```python
from build123d import *

# Parameters (mm, degrees)
SKETCH3_W                                       = 50
SKETCH3_H                                       = 50
BOSS_EXTRUDE1_DEPTH                             = 8
SKETCH3_3_R                                     = 1.5
SKETCH3_3_R_2                                   = 8
CUT_EXTRUDE2_DEPTH                              = 10
SKETCH4_R                                       = 18.5
CUT_EXTRUDE3_DEPTH                              = 4
BOSS_EXTRUDE2_DEPTH                             = 15
BOSS_EXTRUDE2_DEPTH_BACK                        = 23
SKETCH6_W                                       = 80
SKETCH6_H                                       = 5
CSK_FOR_M3_FLAT_HEAD_MACHINE_SCREW1_D           = 3.4
CSK_FOR_M3_FLAT_HEAD_MACHINE_SCREW1_CSINK_D     = 6.3
CSK_FOR_M3_FLAT_HEAD_MACHINE_SCREW1_CSINK_ANGLE = 90
SKETCH11_R                                      = 6.207
SKETCH11_R_2                                    = 5.207
BOSS_EXTRUDE3_DEPTH                             = 5


with BuildPart() as part:
    # Sketch3 → Boss-Extrude1 (new body)
    with BuildSketch(Plane.XY):
        with Locations((0, 25)):
            Rectangle(SKETCH3_W, SKETCH3_H)
    extrude(amount=BOSS_EXTRUDE1_DEPTH)

    # Sketch3_3 → Cut-Extrude2 (cut)
    with BuildSketch(Plane.XY):
        with Locations(Location((-7.75, 38.423393759, 0), (0, 0, 180))):
            Circle(SKETCH3_3_R)
        with Locations(Location((7.75, 38.423393759, 0), (0, 0, 180))):
            Circle(SKETCH3_3_R)
        with Locations(Location((-7.75, 11.576606241, 0), (0, 0, 180))):
            Circle(SKETCH3_3_R)
        with Locations(Location((7.75, 11.576606241, 0), (0, 0, 180))):
            Circle(SKETCH3_3_R)
        with Locations(Location((15.5, 25, 0), (0, 0, 180))):
            Circle(SKETCH3_3_R)
        with Locations(Location((6.062177825, 28.499999999, 0), (0, 0, 180))):
            Circle(SKETCH3_3_R_2)
    extrude(amount=CUT_EXTRUDE2_DEPTH, mode=Mode.SUBTRACT)

    # Sketch4 → Cut-Extrude3 (cut)
    with BuildSketch(Plane.XY.offset(8)):
        with Locations((0, 25)):
            Circle(SKETCH4_R)
    extrude(amount=-CUT_EXTRUDE3_DEPTH, mode=Mode.SUBTRACT)

    # Sketch6 → Boss-Extrude2 (add, two sides: drawn at the far end of the back side and taken through both)
    with BuildSketch(Plane.XY.offset(8).offset(-BOSS_EXTRUDE2_DEPTH_BACK)):
        with Locations((0, 2.5)):
            Rectangle(SKETCH6_W, SKETCH6_H)
    extrude(amount=BOSS_EXTRUDE2_DEPTH + BOSS_EXTRUDE2_DEPTH_BACK)

    # CSK for M3 Flat Head Machine Screw1 (through all)
    with Locations(Plane(origin=(0, 5, 0), x_dir=(1, 0, 0), z_dir=(0, 1, 0))):
        with Locations((-32.5, 7.5), (-32.5, -15.5), (32.5, -15.5), (32.5, 7.5)):
            CounterSinkHole(CSK_FOR_M3_FLAT_HEAD_MACHINE_SCREW1_D / 2, CSK_FOR_M3_FLAT_HEAD_MACHINE_SCREW1_CSINK_D / 2, counter_sink_angle=CSK_FOR_M3_FLAT_HEAD_MACHINE_SCREW1_CSINK_ANGLE)

    # Sketch11 → Boss-Extrude3 (add)
    with BuildSketch(Plane(origin=(0, 0, 0), x_dir=(-1, 0, 0), z_dir=(0, 0, -1))):
        with Locations((17.917822175, 28.499999999)):
            Circle(SKETCH11_R)
        with Locations((17.917822175, 28.499999999)):
            Circle(SKETCH11_R_2, mode=Mode.SUBTRACT)
    extrude(amount=BOSS_EXTRUDE3_DEPTH)


solid = part.part
```
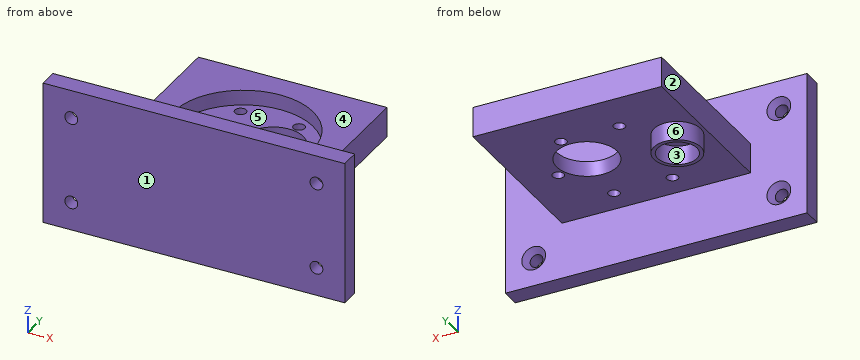
Input: part model. Units: mm. Frame: model coordinates. Face numbers are marked on the shaded views. A direction names the side the tool comes from. Round coordinates to 2 decimals unless told otherwise and drop trailing zeros. Loops run counter-clockwise (first coordinate to the right, second up) from the corner with the lowest first, then second, coordinate; pieces in that order, holes last.
1) Section query B-B on z = 1.5. Return the cut outline in (x, y).
Ans:
outline: (-40, 0) - (40, 0) - (40, 5) - (25, 5) - (25, 50) - (-25, 50) - (-25, 5) - (-40, 5) - close; hole circle Ø3 at (-7.75, 11.58); hole circle Ø3 at (-7.75, 38.42); hole circle Ø16 at (6.06, 28.5); hole circle Ø3 at (7.75, 11.58); hole circle Ø3 at (7.75, 38.42); hole circle Ø3 at (15.5, 25)
2) Pull-direction query (Y, two-part tool) for the marked faces 1, 2 and 3; classes: released by +Y, released by -Y, zero draft, split by the parting line, or undercut.
Ans:
face 1: released by -Y
face 2: zero draft
face 3: undercut
3) Section query C-C on y = 25. Return the cut outline in (x, z), plus the area to 3 significant figures.
Ans:
outline: (-25, 0) - (-23.04, 0) - (-23.04, -5) - (-21.77, -5) - (-21.77, 0) - (-14.06, 0) - (-14.06, -5) - (-12.79, -5) - (-12.79, 0) - (-1.13, 0) - (-1.13, 4) - (-18.5, 4) - (-18.5, 8) - (-25, 8) - close; (13.26, 0) - (14, 0) - (14, 4) - (13.26, 4) - close; (17, 0) - (25, 0) - (25, 8) - (18.5, 8) - (18.5, 4) - (17, 4) - close
area: 195 mm2
4) Pin query (flat end, axial travel): pin 1 (12 mm diameter, centred on y = 28.5, z = -6.5, fed in from +X); pin 2 (9 mm diameter, centred on y = 16.5, z = 2.5, fed in from +X); pin 3 (9.5 mm diameter, centred on x = -17.92, y = 28.5, fed in from -Z); pin 4 (2 mm diameter, centred on x = -32.5, z = 15.5, fed in from +Y). Return the tip coordinate at first contact, or that it passes through.
Ans:
pin 1: stops at x = -11.71
pin 2: stops at x = 25
pin 3: stops at z = 0
pin 4: passes through
5) Section query D-D on x = 7.75. Return the cut outline in (y, z), plus the area to 3 significant figures.
Ans:
outline: (0, -15) - (5, -15) - (5, 0) - (10.08, 0) - (10.08, 4) - (8.2, 4) - (8.2, 8) - (5, 8) - (5, 23) - (0, 23) - close; (13.08, 0) - (20.68, 0) - (20.68, 4) - (13.08, 4) - close; (36.32, 0) - (36.92, 0) - (36.92, 4) - (36.32, 4) - close; (39.92, 0) - (50, 0) - (50, 8) - (41.8, 8) - (41.8, 4) - (39.92, 4) - close
area: 329 mm2
6) Section query A-A on x = -32.5. Return the cut outline in (y, z).
Ans:
outline: (0, -15) - (5, -15) - (5, -10.65) - (3.55, -9.2) - (0, -9.2) - close; (0, -5.8) - (3.55, -5.8) - (5, -4.35) - (5, 12.35) - (3.55, 13.8) - (0, 13.8) - close; (0, 17.2) - (3.55, 17.2) - (5, 18.65) - (5, 23) - (0, 23) - close
7) Set-up query: the marked faces 4, 5 and 6. Return all of +Z, -Z, +X, -X, +Y, -Y with unobstructed straight access to the full face (end or side cutting, diameter ignored); none if empty.
Ans:
face 4: +Z, +X, -X, +Y
face 5: +Z
face 6: -Z
8) Material intervals for line 1 (Y direction, x = -7.75, z = 1); line 2 (Z direction, x = 32.5, y = 2.5); line 3 (X direction, y = 24.5, z = 6.5), sorted ascending.
Ans:
line 1: y = 0 to 10.08, 13.08 to 36.92, 39.92 to 50
line 2: z = -15 to -9.2, -5.8 to 13.8, 17.2 to 23
line 3: x = -25 to -18.49, 18.49 to 25
